```python
from build123d import *

# Parameters (mm, degrees)
SKETCH1_R                 = 6.35
BOSS_EXTRUDE1_DEPTH       = 15
SKETCH2_R                 = 3.1
CUT_EXTRUDE1_DEPTH        = 10
SKETCH3_R                 = 4.1
CUT_EXTRUDE2_DEPTH        = 5
F_6_32_TAPPED_HOLE1_D     = 2.7051
F_6_32_TAPPED_HOLE1_DEPTH = 7
F_6_32_TAPPED_HOLE1_TIP   = 0.81269403
F_6_32_TAPPED_HOLE2_D     = 2.7051
SKETCH14_R                = 12.660953714
BOSS_EXTRUDE2_DEPTH       = 6.35
F_6_32_TAPPED_HOLE3_D     = 2.7051


with BuildPart() as part:
    # Sketch1 → Boss-Extrude1 (new body)
    with BuildSketch(Plane(origin=(0, 0, 0), x_dir=(0, 0, -1), z_dir=(0, -1, 0))):
        Circle(SKETCH1_R)
    extrude(amount=BOSS_EXTRUDE1_DEPTH)

    # Sketch2 → Cut-Extrude1 (cut)
    with BuildSketch(Plane(origin=(0, 0, 0), x_dir=(1, 0, 0), z_dir=(0, 1, 0))):
        Circle(SKETCH2_R)
    extrude(amount=-CUT_EXTRUDE1_DEPTH, mode=Mode.SUBTRACT)

    # Sketch3 → Cut-Extrude2 (cut)
    with BuildSketch(Plane.XZ.offset(15)):
        Circle(SKETCH3_R)
    extrude(amount=-CUT_EXTRUDE2_DEPTH, mode=Mode.SUBTRACT)

    # #6-32 Tapped Hole1
    with Locations(Plane(origin=(-6.349702391, -3.685069286, 0.061478042), x_dir=(-0.009681581, 0, -0.999953132), z_dir=(-0.999953132, 0, 0.009681581))):
        with Locations((0, 0)):
            Hole(F_6_32_TAPPED_HOLE1_D / 2, depth=F_6_32_TAPPED_HOLE1_DEPTH)
            with Locations((0, 0, -(F_6_32_TAPPED_HOLE1_DEPTH + F_6_32_TAPPED_HOLE1_TIP / 2))):  # 118° drill point
                Cone(0, F_6_32_TAPPED_HOLE1_D / 2, F_6_32_TAPPED_HOLE1_TIP, mode=Mode.SUBTRACT)

    # #6-32 Tapped Hole2 (through all)
    with Locations(Plane(origin=(-6.349688123, -12.545322132, 0.062934409), x_dir=(-0.009910931, 0, -0.999950886), z_dir=(-0.999950886, 0, 0.009910931))):
        with Locations((0, 0)):
            Hole(F_6_32_TAPPED_HOLE2_D / 2)

    # Sketch14 → Boss-Extrude2 (add)
    with BuildSketch(Plane(origin=(0, 0, 0), x_dir=(1, 0, 0), z_dir=(0, 1, 0))):
        Circle(SKETCH14_R)
    extrude(amount=BOSS_EXTRUDE2_DEPTH)

    # #6-32 Tapped Hole3 (through all)
    with Locations(Plane(origin=(0, 0, 0), x_dir=(-1, 0, 0), z_dir=(0, -1, 0))):
        with Locations((-9.779, 0), (0, 9.779), (9.779, 0), (0, -9.779)):
            Hole(F_6_32_TAPPED_HOLE3_D / 2)


solid = part.part
```
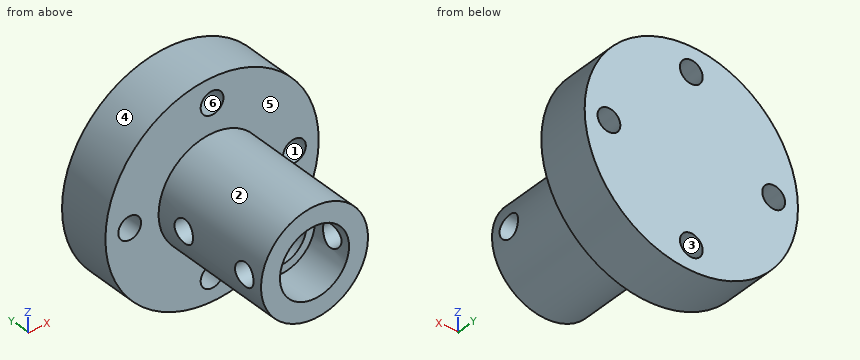
Work out the finished part from the listing and answer in its coordinate system (mm). Face numbers are marked on the shaded views. A direction names the side the tool comes from. Round coordinates to 2 decimals unless told otherwise and drop trailing zeros. Loops run counter-clockwise (first coordinate to the right, second up) from the corner with the lowest first, then second, coordinate; pieces in that order, holes last.
(1) The part is cut by section B-B, the plane z = -10.75. Give the vertices of the cut face in (x, y), and give its area (3 significant figures).
Computed values:
outline: (-6.69, 0) - (-0.94, 0) - (-0.94, 6.35) - (-6.69, 6.35) - close; (0.94, 0) - (6.69, 0) - (6.69, 6.35) - (0.94, 6.35) - close
area: 73.0 mm2
(2) Each of these flat-tipped pins is pushed along its axis until it touches: P1, Ø4.5, axis at x = 0, z = -9.779, coming from the -Y side; P2, Ø6.5, axis at x = -1, z = 0.5, coming from the -Y side; P3, Ø10, axis at x = 10, y = 3.5, coming from the +Z side. Where does it stop, or does it pass through?
Computed values:
P1: stops at y = 0
P2: stops at y = -15
P3: stops at z = 11.63
(3) The part is cut by section A-A, the plane x = 0. Give the vertices of the cut face in (y, z), and give its area (3 significant figures).
Computed values:
outline: (-15, -6.35) - (0, -6.35) - (0, -8.43) - (6.35, -8.43) - (6.35, 8.43) - (0, 8.43) - (0, 6.35) - (-15, 6.35) - (-15, 4.1) - (-10, 4.1) - (-10, 3.1) - (0, 3.1) - (0, -3.1) - (-10, -3.1) - (-10, -4.1) - (-15, -4.1) - close; (0, -12.66) - (6.35, -12.66) - (6.35, -11.13) - (0, -11.13) - close; (0, 11.13) - (6.35, 11.13) - (6.35, 12.66) - (0, 12.66) - close
area: 214 mm2
(4) The mould has two halves that part along Z. Classify the marked faces 3, 4, 5 and 6: pulls with the +Z half, pulls with the -Z half, needs draft (parallel to the pull), parting line crosses it, or undercut.
Computed values:
face 3: undercut
face 4: parting line crosses it
face 5: needs draft
face 6: undercut
(5) For the marked faces 1 and 2, determine the directions among +Z, -Z, +X, -X, +Y, -Y from which every point of the face is accessible in a straight line to the end or side of a thin tool.
Computed values:
face 1: +Y, -Y
face 2: -Y
(6) Find the intervals of material crossed by L1, parallel to Z at x = 0, y = 3.75; L2, parallel to X at y = -2, z = 0; L3, parallel to Y at x = -4.5, z = -11, in increasing order.
Computed values:
L1: z = -12.66 to -11.13, -8.43 to 8.43, 11.13 to 12.66
L2: x = -6.35 to -3.1, 3.1 to 6.35
L3: y = 0 to 6.35
(7) The part is cut by section C-C, the plane y = 2.75. Give the vertices of the cut face in (x, z), and give its area (3 significant figures).
Computed values:
outline: circle Ø25.32 at (0, 0); hole circle Ø2.71 at (-9.78, 0); hole circle Ø2.71 at (0, -9.78); hole circle Ø2.71 at (0, 9.78); hole circle Ø2.71 at (9.78, 0)
area: 481 mm2
(8) The part is cut by section D-D, the plane z = -3.75. Give the vertices of the cut face in (x, y).
Computed values:
outline: (-12.09, 0) - (-5.12, 0) - (-5.12, -15) - (-1.66, -15) - (-1.66, -10) - (1.66, -10) - (1.66, -15) - (5.12, -15) - (5.12, 0) - (12.09, 0) - (12.09, 6.35) - (-12.09, 6.35) - close
